```python
from build123d import *

# Parameters (mm, degrees)
BOSS_EXTRU_1_DEPTH      = 10
BOSS_EXTRU_1_DEPTH_BACK = 10
ESQUISSE2_R             = 5
ENL_V_MAT_EXTRU_1_DEPTH = 10
ESQUISSE3_R             = 5
ENL_V_MAT_EXTRU_2_DEPTH = 10


with BuildPart() as part:
    # Esquisse1 → Boss.-Extru.1 (new, two sides: drawn at the far end of the back side and taken through both)
    with BuildSketch(Plane.XY.offset(-BOSS_EXTRU_1_DEPTH_BACK)):
        Polygon((0, 0), (10, 0), (10, 20), (60, 20), (60, 30), (0, 30), align=None)
    extrude(amount=BOSS_EXTRU_1_DEPTH + BOSS_EXTRU_1_DEPTH_BACK)

    # Esquisse2 → Enl_v. mat.-Extru.1 (cut)
    with BuildSketch(Plane.XZ.offset(-20)):
        with Locations(Location((50, 0, 0), (0, 0, 270))):
            Circle(ESQUISSE2_R)
    extrude(amount=-ENL_V_MAT_EXTRU_1_DEPTH, mode=Mode.SUBTRACT)

    # Esquisse3 → Enl_v. mat.-Extru.2 (cut)
    with BuildSketch(Plane.ZY):
        with Locations((0, 6)):
            Circle(ESQUISSE3_R)
    extrude(amount=-ENL_V_MAT_EXTRU_2_DEPTH, mode=Mode.SUBTRACT)


solid = part.part
```
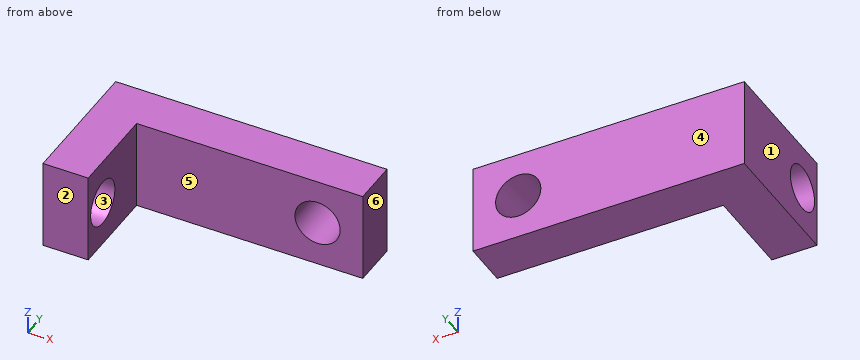
Build history of the part. All positions in model axes, mm. Face numbers are marked on the shaded views. A direction names the side the tool comes from. Round coordinates to 2 decimals unless told otherwise and drop trailing zeros. Write each loop counter-clockwise with the first axis right and the second up, starting at its lowest first coordinate (ties: lowest second). Pieces come first, ordered by that corner, then holes.
1) Pin check, flat tips, straight feed: pin 1 (8 mm diameter, centred on x = 20, z = 7, fed in from -Y); pin 2 (6 mm diameter, centred on x = 7.5, z = 7.5, fed in from -Y); pin 3 (1 mm diameter, centred on x = 26, y = 18, fed in from +Z); pin 4 (12 mm diameter, centred on y = 9.5, z = 5, fed in from +X). Stop position of each tip, or through.
2) Band-saw the part on B-B, the plane z = 0. List the corners of the cut face in (x, y), and give its area (3 significant figures).
3) Drill centre lines: probe 1 along Y at (x, z) = (2.75, 0); probe 2 along Y at (x, z) = (36, -6.25); probe 3 along X at (y, z) = (27.5, 0). Where is each one in solid material? Low to high.
4) 3-axis set-ups, long thin cutter, end or side, ignore diameter. For the marked faces 5 and 6: which of +Z, -Z, +X, -X, +Y, -Y reach the whole face in a straight line?
5) Band-saw the part on A-A, the plane y = 6. List the corners of the cut face in (x, z).
6) Mould opens along Y. For the marked faces 1, 2, 3 and 4 say: +Y half, -Y half, draft (parallel to the pull), parting line (faces both ways), or undercut.
7) Band-saw the part on C-C, the plane x = 50. List the corners of the cut face in (y, z).
8) Band-saw the part on D-D, the plane y = 26.25. List the corners of the cut face in (x, z).
Ans:
1. pin 1: stops at y = 20
1. pin 2: stops at y = 0
1. pin 3: passes through
1. pin 4: stops at x = 10
2. outline: (0, 0) - (10, 0) - (10, 1) - (0, 1) - close; (0, 11) - (10, 11) - (10, 20) - (45, 20) - (45, 30) - (0, 30) - close; (55, 20) - (60, 20) - (60, 30) - (55, 30) - close
2. area: 600 mm2
3. probe 1: y = 0 to 1, 11 to 30
3. probe 2: y = 20 to 30
3. probe 3: x = 0 to 45, 55 to 60
4. face 5: +Z, -Z, +X, -Y
4. face 6: +Z, -Z, +X, +Y, -Y
5. outline: (0, -10) - (10, -10) - (10, -5) - (0, -5) - close; (0, 5) - (10, 5) - (10, 10) - (0, 10) - close
6. face 1: draft
6. face 2: -Y half
6. face 3: undercut
6. face 4: +Y half
7. outline: (20, -10) - (30, -10) - (30, -5) - (20, -5) - close; (20, 5) - (30, 5) - (30, 10) - (20, 10) - close
8. outline: (0, -10) - (60, -10) - (60, 10) - (0, 10) - close; hole circle Ø10 at (50, 0)
